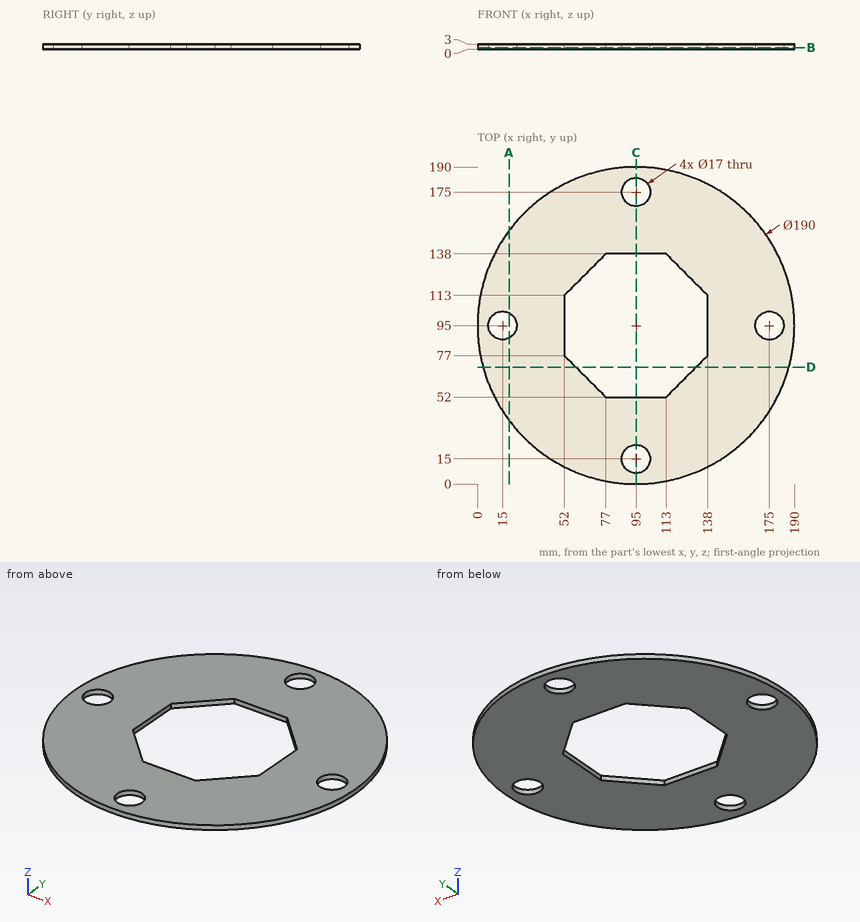
Study the drawing (mm; zero at the part's minimum x, y, z) and answer. Coordinates: 2 decimals unless noted, no trailing zeros. Write each loop counter-clockwise with the first axis right and the second up, starting at its lowest first coordinate (ties: lowest second). Pieces come first, ordered by that corner, then holes.
Q1. A cutting plane is placed at D-D, the plane y = 70. Give the vertices of the cut face in (x, z), then the cut area to 3 significant figures.
Q2. A cutting plane is placed at C-C, the plane x = 95. Give the vertices of the cut face in (y, z).
Q3. A cutting plane is placed at B-B, the plane z = 0.9. Give the vertices of the cut face in (x, y), then the cut area to 3 significant figures.
Q4. A cutting plane is placed at A-A, the plane x = 19. Give the vertices of the cut face in (y, z), then the cut area to 3 significant figures.
Q5. Each of these flat-tipped pins is pushed along its axis until it touches: pin 1 Ø1 at (y, z) = (170.5, 2) entering from +X; pin 2 Ø1.5 at (x, z) = (39.5, 2.5) entering from -Y; pin 3 Ø0.9 at (x, z) = (101.5, 1.5) entering from +Y. Where does it stop, or does it pass through?
Q6. Find the intervals of material crossed by line 1 (Y direction, x = 95, z = 0.95); line 2 (X direction, y = 92.5, z = 2.45); line 3 (Y direction, x = 15, z = 1.3), in increasing order.
Findings below:
1. outline: (3.35, 0) - (59, 0) - (59, 3) - (3.35, 3) - close; (131, 0) - (186.65, 0) - (186.65, 3) - (131, 3) - close
1. area: 334 mm2
2. outline: (0, 0) - (6.5, 0) - (6.5, 3) - (0, 3) - close; (23.5, 0) - (52, 0) - (52, 3) - (23.5, 3) - close; (138, 0) - (166.5, 0) - (166.5, 3) - (138, 3) - close; (183.5, 0) - (190, 0) - (190, 3) - (183.5, 3) - close
3. outline: circle Ø190 at (95, 95); hole circle Ø17 at (15, 95); hole (52, 77) - (77, 52) - (113, 52) - (138, 77) - (138, 113) - (113, 138) - (77, 138) - (52, 113) - close; hole circle Ø17 at (95, 15); hole circle Ø17 at (95, 175); hole circle Ø17 at (175, 95)
3. area: 21,300 mm2
4. outline: (38, 0) - (87.5, 0) - (87.5, 3) - (38, 3) - close; (102.5, 0) - (152, 0) - (152, 3) - (102.5, 3) - close
4. area: 297 mm2
5. pin 1: stops at x = 153.31
5. pin 2: stops at y = 17.36
5. pin 3: stops at y = 189.81
6. line 1: y = 0 to 6.5, 23.5 to 52, 138 to 166.5, 183.5 to 190
6. line 2: x = 0.03 to 6.88, 23.12 to 52, 138 to 166.88, 183.12 to 189.97
6. line 3: y = 43.77 to 86.5, 103.5 to 146.23
